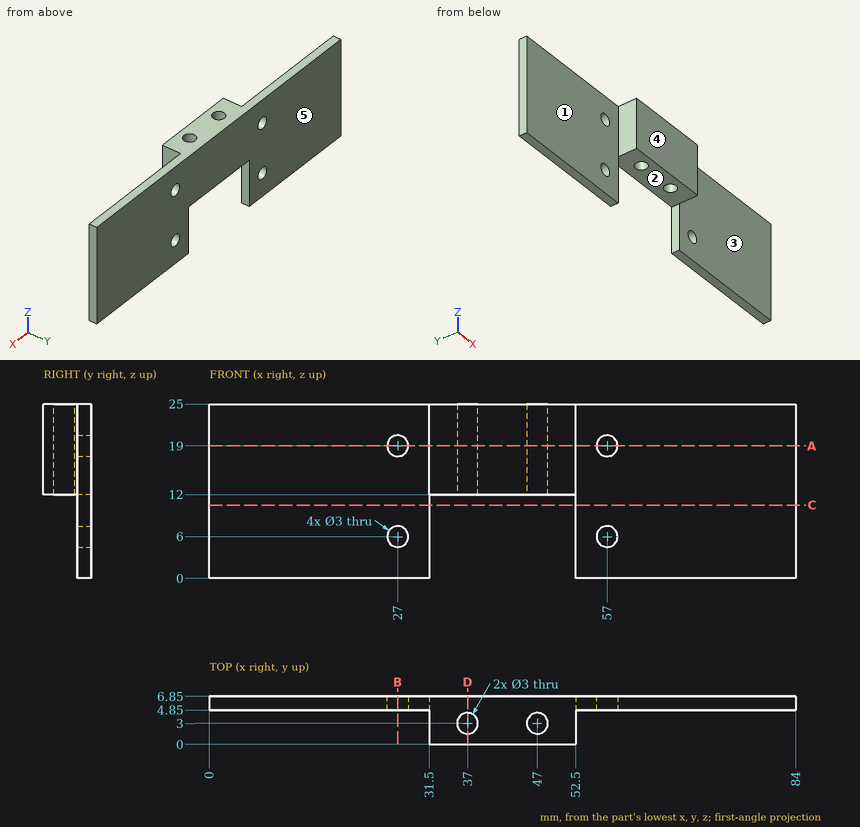
Check sheet for the drawn part. Datum: minimum x, y, z corner. Units: mm. A direction names the side the tool comes from. Coordinates: 2 decimals unless noted, no trailing zeros. Order: outer loops, then holes, each group sorted by start corner. A loop starts at its lowest first (then second) coordinate and runs counter-clockwise, first axis right, second up. Notation, with made-up numbers: M 26.25,61 L 35.25,61 A20 cw 35.25,65 Z; hole C 9.25,6.25 d5. An arc over 180 degrees is marked long. One line per question, with ' | ' between items. Start each with the question number.
Item 1: Cross-section at D-D on x = 37. Enter the section's corners in (y, z).
Item 2: Cross-section at C-C on z = 10.5. Enter the section's corners in (x, y).
Item 3: Set-up check for the marked faces 1, 2, 3, 4 and 5: record each of +Z, -Z, +X, -X, +Y, -Y from which the full face is reachable in a straight line by a thin tool's end or side.
Item 4: Cross-section at B-B on x = 27. Enter the section's corners in (y, z).
Item 5: Gauge pin test, flat ends, axial feed: pin 1 (4 mm diameter, centred on x = 70, y = 2.5, fed in from +Z); pin 2 (1.5 mm diameter, centred on y = 2.5, z = 21.5, fed in from -X); pin 3 (1.5 mm diameter, centred on y = 4, z = 15.5, fed in from +X); pin 4 (3.5 mm diameter, centred on x = 47, y = 3, fed in from -Z). Record the tip position at first contact, or that the pin passes through.
Item 6: Material ranges on L1, parallel to Z at x = 27, y = 5.5; L2, parallel to Z at x = 58, y = 6.5; L3, parallel to Y at x = 47, z = 19.5, recorded low to high. Write a range as [from, to].
Item 7: Cross-section at A-A on z = 19. Enter the section's corners in (x, y), then the cut area to 3 significant figures.
Findings:
1) outline: M 0,12 L 1.5,12 L 1.5,25 L 0,25 Z; M 4.5,12 L 6.85,12 L 6.85,25 L 4.5,25 Z
2) outline: M 0,4.85 L 31.5,4.85 L 31.5,6.85 L 0,6.85 Z; M 52.5,4.85 L 84,4.85 L 84,6.85 L 52.5,6.85 Z
3) face 1: +Z, -Z, -X, -Y | face 2: -Z, +Y, -Y | face 3: +Z, -Z, +X, -Y | face 4: +Z, -Z, +X, -X, -Y | face 5: +Z, -Z, +X, -X, +Y
4) outline: M 4.85,0 L 6.85,0 L 6.85,4.5 L 4.85,4.5 Z; M 4.85,7.5 L 6.85,7.5 L 6.85,17.5 L 4.85,17.5 Z; M 4.85,20.5 L 6.85,20.5 L 6.85,25 L 4.85,25 Z
5) pin 1: passes through | pin 2: stops at x = 31.5 | pin 3: stops at x = 52.5 | pin 4: stops at z = 12
6) L1: z = [0, 4.5], [7.5, 17.5], [20.5, 25] | L2: z = [0, 4.88], [7.12, 17.88], [20.12, 25] | L3: y = [0, 1.5], [4.5, 6.85]
7) outline: M 0,4.85 L 25.5,4.85 L 25.5,6.85 L 0,6.85 Z; M 28.5,4.85 L 31.5,4.85 L 31.5,0 L 52.5,0 L 52.5,4.85 L 55.5,4.85 L 55.5,6.85 L 28.5,6.85 Z; M 58.5,4.85 L 84,4.85 L 84,6.85 L 58.5,6.85 Z; hole C 37,3 d3; hole C 47,3 d3 | area: 244 mm²
